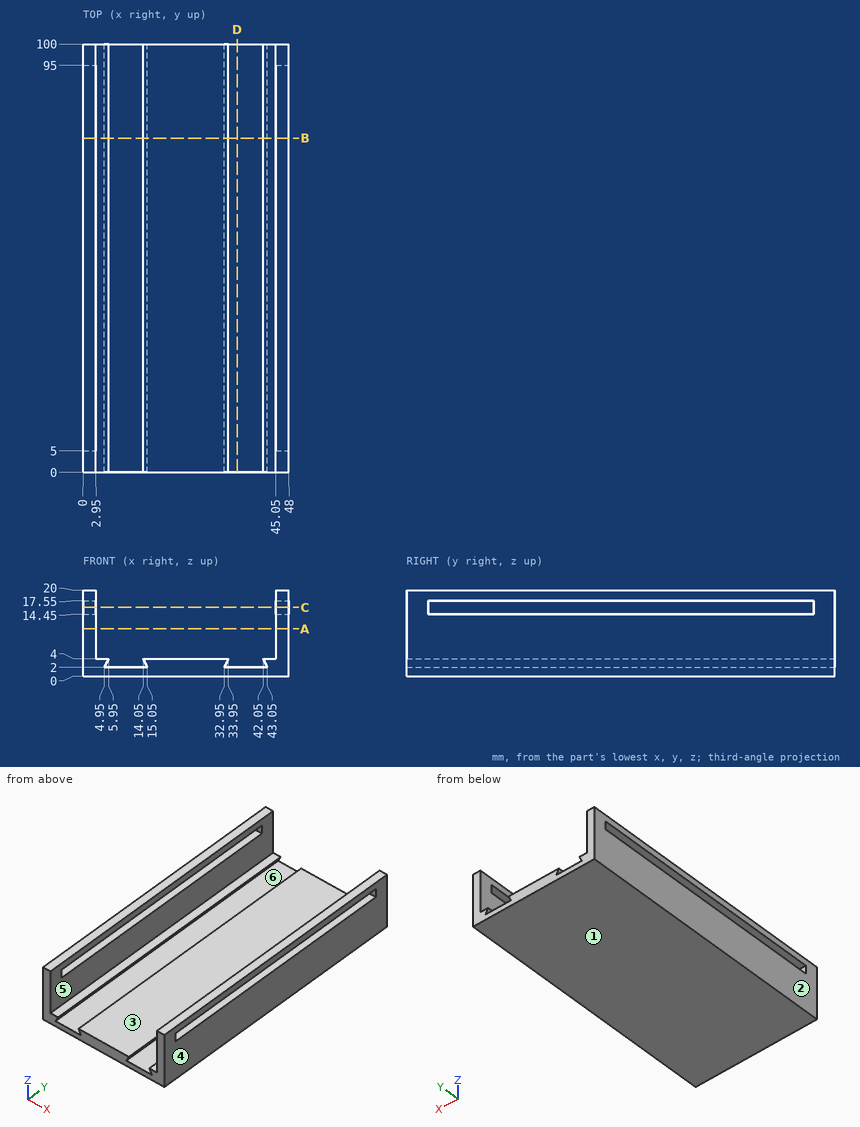
For this review, use the dimensioned drawing (mm, ordinates from the lowest corner) and the shaded views. A direction names the side the tool comes from. Round coordinates to 2 decimals unless told otherwise and drop trailing zeros. Write each loop counter-clockwise with the first axis right and the second up, starting at its lowest first coordinate (ties: lowest second). Pieces come first, ordered by that corner, then holes. Notation, with made-up numbers: (51.25, 39.25) - (93.25, 39.25) arc R30 cw to (93.25, 64.25) - close; hole circle Ø1 at (5, 54.5). An arc over 180 degrees is marked (long way). One line per item, written item: value. Start each with the question number.
1. Machinability: for the marked faces 4, 5 and 6, which of the approach directions +Z, -Z, +X, -X, +Y, -Y give a long, thin tool a straight path to every point of the face, cutting with its end or side? Answer none if there is none.
2. To check wall thickness, follow L1, parallel to X at y = 57, z = 10.5; L2, parallel to Z at x = 2, y = 16.5; L3, parallel to Z at x = 35.5, y = 39.5. State the ranges of each line that lie inside material, in increasing order. Write a range as from..to.
3. Consider section C-C on z = 16. Write out the cut boundary in (x, y).
4. Consider section A-A on z = 11. Write out the cut boundary in (x, y).
5. The part is to be moulded in two halves that separate along X. For the marked faces 1, 2 and 3, say which applies: released by +X, released by -X, zero draft, split by the parting line, or undercut.
6. Clearance check with flat-ended pins moving along their axes: P1, Ø11, axis at x = 9.5, y = 31, coming from the +Z side; P2, Ø1, axis at x = 29, y = 88.5, coming from the -Z side; P3, Ø3, axis at x = 39, y = 54, coming from the +Z side; P4, Ø12, axis at x = 18, z = 14.5, coming from the -Y side. State where each tip first meets the part, or that it passes through.
7. Consider section B-B on y = 78. Write out the cut boundary in (x, z).
8. Consider section D-D on x = 36. Write out the cut boundary in (y, z).
Checks:
1. face 4: +Z, -Z, +X, +Y, -Y
1. face 5: +Z, +Y, -Y
1. face 6: +Y, -Y
2. L1: x = 0..2.95, 45.05..48
2. L2: z = 0..14.45, 17.55..20
2. L3: z = 0..2
3. outline: (0, 0) - (2.95, 0) - (2.95, 5) - (0, 5) - close; (0, 95) - (2.95, 95) - (2.95, 100) - (0, 100) - close; (45.05, 0) - (48, 0) - (48, 5) - (45.05, 5) - close; (45.05, 95) - (48, 95) - (48, 100) - (45.05, 100) - close
4. outline: (0, 0) - (2.95, 0) - (2.95, 100) - (0, 100) - close; (45.05, 0) - (48, 0) - (48, 100) - (45.05, 100) - close
5. face 1: zero draft
5. face 2: released by -X
5. face 3: undercut
6. P1: stops at z = 4
6. P2: stops at z = 0
6. P3: stops at z = 2
6. P4: passes through
7. outline: (0, 0) - (48, 0) - (48, 14.45) - (45.05, 14.45) - (45.05, 4) - (42.05, 4) - (43.05, 2) - (32.95, 2) - (33.95, 4) - (14.05, 4) - (15.05, 2) - (4.95, 2) - (5.95, 4) - (2.95, 4) - (2.95, 14.45) - (0, 14.45) - close; (0, 17.55) - (2.95, 17.55) - (2.95, 20) - (0, 20) - close; (45.05, 17.55) - (48, 17.55) - (48, 20) - (45.05, 20) - close
8. outline: (0, 0) - (100, 0) - (100, 2) - (0, 2) - close
